```python
from build123d import *

# Parameters (mm, degrees)
F1_W       = 185.7
F1_H       = 97.25
F2_DEPTH   = 72
F2_FACE_W  = 72
F2_FACE_H  = 97.25
F4_W       = 72
F4_H       = 97.25
F6_R       = 25
F2_FACE1_W = 72
F2_FACE1_H = 97.25
F8_W       = 48.5
F8_H       = 97.25
F10_R      = 3.75
F11_DEPTH  = 12.5


with BuildPart() as f2:
    # F1 (on offset) → F2 (new body)
    with BuildSketch(Plane.XZ.offset(-84.5)):
        Rectangle(F1_W, F1_H)
    extrude(amount=F2_DEPTH)

    # F2_face (on face) → F5 section 0
    with BuildSketch(Plane(origin=(-92.85, 48.5, 0), x_dir=(0, -1, 0), z_dir=(-1, 0, 0))):
        Rectangle(F2_FACE_W, F2_FACE_H)
    # F4 (on offset) → F5 section 1
    with BuildSketch(Plane(origin=(-117.85, 0, 0), x_dir=(0, -1, 0), z_dir=(-1, 0, 0))):
        with Locations((-48.5, 0)):
            Rectangle(F4_W, F4_H)
    loft()

    # F6
    f6_edges = [f2.edges().sort_by_distance(p)[0] for p in [
        (-117.85, 84.5, 0),
        (-117.85, 12.5, 0),
        (-117.85, 48.5, 48.625),
        (-117.85, 48.5, -48.625),
    ]]
    fillet(f6_edges, radius=F6_R)

    # F2_face1 (on face) → F9 section 0
    with BuildSketch(Plane(origin=(92.85, 48.5, 0), x_dir=(0, 1, 0), z_dir=(1, 0, 0))):
        Rectangle(F2_FACE1_W, F2_FACE1_H)
    # F8 (on offset) → F9 section 1
    with BuildSketch(Plane.YZ.offset(143.15)):
        with Locations((36.75, 0)):
            Rectangle(F8_W, F8_H)
    loft()

    # F10 (on face) → F11 (join)
    with BuildSketch(Plane.XZ.offset(-12.5)):
        with Locations((-67.35, -28.875)):
            Circle(F10_R)
        with Locations((50.15, -28.875)):
            Circle(F10_R)
        with Locations((50.15, 28.875)):
            Circle(F10_R)
        with Locations((-67.35, 28.875)):
            Circle(F10_R)
    extrude(amount=F11_DEPTH)


solid = f2.part
```
Geometry: final body of the model. Coordinates: model frame, mm. A direction names the side the tool comes from. Round coordinates to 2 decimals unless told otherwise and drop trailing zeros. Order: outer loops, then holes, each group sorted by start corner. A loop starts at its lowest first (then second) coordinate and runs counter-clockwise, first axis right, second up. Notation, with made-up numbers: (-15, 37) - (18, 37) arc R8 ccw to (18, 44) - close; hole circle Ø2 at (10.5, 65.5). An arc over 180 degrees is marked (long way). Write item = value, one per line. Start each with the question number.
Q1. Cut plane C-C on x = -5.5. Return the cut outline in (y, z) (3 decimals).
Q2. Pull-direction query (X, two-part tool) for faces 3 (the flat face through (22, 49, 48.625)), 4 (the cylindrical face through (53.727, 6.338, -27.749)), 5 (the cylindrical face through (-106.963, 80.135, 0.681)); classes: +X half, -X half, draft (parallel to the pull), parting line (faces both ways), or undercut.
Q3. Cut plane A-A on z = -20. Return the cut outline in (x, y).
Q4. Ray query, line 1 (Y direction, x = 12, z = 39.5); line 2 (Z direction, x = 52, y = 12); line 3 (Z direction, x = 47.5, y = 8.5). Return the intervals inside material, ascending. Write a range as from..to.
Q5. Access query for faces 1 (the flat face through (143.15, 36, 0)), 2 (the cylindrical face through (-71.096, 6.338, -28.71)). Directions: +Z, -Z, +X, -X, +Y, -Y. A direction counts if a zero-diameter tool reaches every point of the face in a straight line with its end or side. Return the directions, or none.
Q6. Cut plane B-B on x = 50.15. Return the cut outline in (y, z) (3 decimals).
Q7. Pin query (flat end, axial travel): pin 1 (2 mm diameter, centred on y = 72, z = 20.5, fed in from +X); pin 2 (12 mm diameter, centred on x = -12, z = 23, fed in from -Y); pin 3 (10 mm diameter, centred on y = 66, z = 26, fed in from -X). Return the tip coordinate at first contact, or that it passes through.
Outcome:
q1.outline = (12.5, -48.625) - (84.5, -48.625) - (84.5, 48.625) - (12.5, 48.625) - close
q2.face_3 = draft
q2.face_4 = undercut
q2.face_5 = -X half
q3.outline = (-117.85, 37.5) arc R25 ccw to (-92.85, 12.5) - (143.15, 12.5) - (143.15, 61) - (92.85, 84.5) - (-92.85, 84.5) arc R25 ccw to (-117.85, 59.5) - close
q4.line_1 = 12.5..84.5
q4.line_2 = -32.14..-25.61, 25.61..32.14
q4.line_3 = -31.53..-26.22, 26.22..31.53
q5.face_1 = +Z, -Z, +X, +Y, -Y
q5.face_2 = -Y
q6.outline = (0, -32.625) - (12.5, -32.625) - (12.5, -48.625) - (84.5, -48.625) - (84.5, 48.625) - (12.5, 48.625) - (12.5, 32.625) - (0, 32.625) - (0, 25.125) - (12.5, 25.125) - (12.5, -25.125) - (0, -25.125) - close
q7.pin_1 = 121.75
q7.pin_2 = 12.5
q7.pin_3 = -117.8
